Check sheet for the modelled part. Datum: model origin and axes. Units: mm. A direction names the side the tool comes from. Give positions to 0.01 mm unless a question says otherwise; leave off trailing zeros. Loops run counter-clockwise (first coordinate to the right, second up) from the corner with the lowest first, then second, coordinate; pieces in that order, holes last. Notation, with made-up numbers: M -31.75,89.25 L -7.75,89.25 A9 ccw -7.75,99.25 Z; hole C 65,70 d11. An arc over 180 degrees is marked long. One line per question, with ' | ' between items. Start each with the question number.
from build123d import *

# Parameters (mm, degrees)
SKETCH1_R           = 8.255
BOSS_EXTRUDE1_DEPTH = 33.3756
SKETCH2_R           = 3.048
BOSS_EXTRUDE2_DEPTH = 0.508
SKETCH3_R           = 5.08
BOSS_EXTRUDE3_DEPTH = 0.1016
FILLET1_R           = 0.508
FILLET2_R           = 0.254


with BuildPart() as part:
    # Sketch1 → Boss-Extrude1 (new body)
    with BuildSketch(Plane(origin=(0, 0, 0), x_dir=(1, 0, 0), z_dir=(0, 1, 0))):
        Circle(SKETCH1_R)
    extrude(amount=BOSS_EXTRUDE1_DEPTH)

    # Sketch2 → Boss-Extrude2 (add)
    with BuildSketch(Plane(origin=(0, 33.3756, 0), x_dir=(1, 0, 0), z_dir=(0, 1, 0))):
        Circle(SKETCH2_R)
    extrude(amount=BOSS_EXTRUDE2_DEPTH)

    # Sketch3 → Boss-Extrude3 (add)
    with BuildSketch(Plane.XZ):
        Circle(SKETCH3_R)
    extrude(amount=BOSS_EXTRUDE3_DEPTH)

    # Fillet1
    fillet1_edges = [part.edges().sort_by_distance(p)[0] for p in [
        (-8.255, 0, 0),
        (-8.255, 33.3756, 0),
    ]]
    fillet(fillet1_edges, radius=FILLET1_R)

    # Fillet2
    fillet2_edges = [part.edges().sort_by_distance(p)[0] for p in [
        (-3.048, 33.8836, 0),
    ]]
    fillet(fillet2_edges, radius=FILLET2_R)


solid = part.part
Q1. Depth check by flat-ended pin: P1, Ø6, axis at y = 7, z = -6, coming from the -X side; P2, Ø4, axis at x = -5, y = 22, coming from the +Z side. Enter the tip coordinate at first touch or a pass-through.
Q2. Cross-section at A-A (y = 4). Record the cut outline in (x, z) (3 decimals), and give its area (3 significant figures).
Q3. Material ranges on probe 1 along Y at (x, z) = (-6.25, 1.25); probe 2 along Y at (x, z) = (4.5, -2); probe 3 along Z at (x, y) = (0.75, 9.5), recorded low to high. Write a range as from..to.
Q4. Access from +Z, -Z, +X, -X, +Y, -Y to the whole of each face (thin tool, end or side, straight path). Record for faces 1 (the flat face through (5, 0, 2)), 2 (the flat face through (3.3, 33.376, -0.1)), 3 (the flat face through (0, 33.884, 0)).
Solved:
1) P1: stops at x = -7.69 | P2: stops at z = 7.69
2) outline: C 0,0 d16.51 | area: 214 mm²
3) probe 1: y = 0..33.38 | probe 2: y = -0.1..33.38 | probe 3: z = -8.22..8.22
4) face 1: -Y | face 2: +Y | face 3: +Z, -Z, +X, -X, +Y
